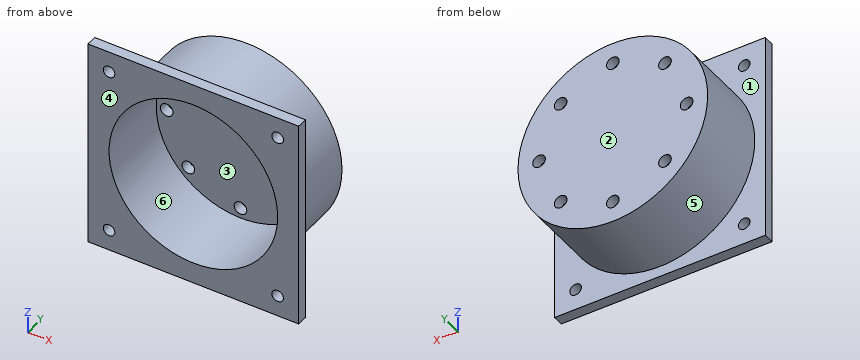
Autodesk Inventor part; units mm, degrees
ref_plane "YZ Plane" through (0, 0, 0) normal (1, 0, 0) x (0, 1, 0)
ref_plane "XZ Plane" through (0, 0, 0) normal (0, 1, 0) x (-1, 0, 0)
ref_plane "XY Plane" through (0, 0, 0) normal (0, 0, 1) x (1, 0, 0)
sketch "Sketch1" plane through (0, 0, 0) normal (0, 1, 0) x (-1, 0, 0)
  line L0 (50, 50) -> (-50, 50)
  line L1 (-50, 50) -> (-50, -50)
  line L2 (-50, -50) -> (50, -50)
  line L3 (50, -50) -> (50, 50)
  circle A0 centre (0, 0) radius 35
  circle A1 centre (40, 40) radius 2.75
  circle A2 centre (-40, 40) radius 2.75
  circle A3 centre (-40, -40) radius 2.75
  circle A4 centre (40, -40) radius 2.75
  point P0 (50, 0)
  point P1 (0, -50)
  dimension "d0" = 100
  dimension "d1" = 100
  dimension "d2" = 70
  dimension "d3" = 5.5
  dimension "d4" = 10
  dimension "d5" = 10
  dimension "d8" = 360
extrude "Extrusion1" add sketch "Sketch1" along normal blind 5
sketch "Sketch2" plane through (0, 0, 0) normal (0, -1, 0) x (1, 0, 0)
  circle A0 centre (0, 0) radius 45
  dimension "d12" = 90
extrude "Extrusion2" cut sketch "Sketch2" against normal blind 10
sketch "Sketch3" plane through (0, 0, 0) normal (0, -1, 0) x (1, 0, 0)
  circle A0 centre (0, 0) radius 45
  circle A1 centre (0, 0) radius 40
  dimension "d15" = 90
  dimension "d16" = 80
extrude "Extrusion3" add sketch "Sketch3" against normal blind 40
sketch "Sketch4" plane through (0, 40, 0) normal (0, 1, 0) x (1, 0, 0)
  circle A0 centre (0, 0) radius 40
extrude "Extrusion4" add sketch "Sketch4" against normal blind 5
sketch "Sketch5" plane through (0, 35, 0) normal (0, -1, 0) x (1, 0, 0)
  circle A0 centre (0, 35) radius 3
  point P0 (0, 0)
  dimension "d21" = 6
  dimension "d22" = 35
extrude "Extrusion5" cut sketch "Sketch5" against normal up to next
pattern_circular "Circular Pattern1" count 8 over 360 about axis through (0, 0, 0) along (0, 1, 0) of "Extrusion5"
properties part number "connector plate"
Could you check a few things on this model? Use its own coordinates, in mm. Face numbers are marked on the shaded views. A direction names the side the tool comes from. Coordinates: 2 decimals unless noted, no trailing zeros. Write each loop counter-clockwise with the first axis right and the second up, starting at its lowest first coordinate (ties: lowest second). Pieces come first, ordered by that corner, then holes. Notation, with made-up numbers: M 7.5,15.25 L 38.5,15.25 A24 cw 38.5,53.25 Z; hole C 74,12 d11. An arc over 180 degrees is marked long. Answer as CSV lines item,"result". Start each with the question number.
1) For the marked faces 1 and 2, which set-ups out of +Z, -Z, +X, -X, +Y, -Y let a thin tool reach every point of the face, with its end or its side?
2) Please list where these lines run through material, in increasing order: line 1 (Z direction, x = 0, y = 38.05); line 2 (Z direction, x = 0, y = 23.5); line 3 (Y direction, x = -2, z = 22). Write a range as from..to.
3) For P1, Ø7, axis at x = 35, z = 0, coming from the -Y side; P2, Ø4, axis at x = -15, y = 23.5, coming from the +Z side; P3, Ø6, axis at x = -18.5, y = 10, coming from the +Z side, each with a flat end and sliding along its axis, tell me the tip position at first contact or that it passes through.
4) We'd pull the mould along Z, two halves only. Please class the marked faces 3, 4, 5 and 6: +Z half, -Z half, draft (parallel to the pull), parting line (faces both ways), or undercut.
5) I want a section at A-A, the plane x = 0. Please give me the cut outline in (y, z).
6) I want a section at D-D, the plane z = -24. Please give me the cut outline in (x, y), and give its area (4 significant figures).
7) I want a section at B-B, the plane z = -35. Please give me the cut outline in (x, y).
8) I want a section at C-C, the plane y = 23. Please give me the cut outline in (x, z).
Data:
1,face 1,"+Y"
1,face 2,"+Z, -Z, +X, -X, +Y"
2,line 1,"z = -45..-38, -32..32, 38..45"
2,line 2,"z = -45..-40, 40..45"
2,line 3,"y = 35..40"
3,P1,"stops at y = 35"
3,P2,"stops at z = 43.08"
3,P3,"stops at z = 42.25"
4,face 3,"undercut"
4,face 4,"draft"
4,face 5,"parting line"
4,face 6,"undercut"
5,outline,"M 0,-50 L 5,-50 L 5,-45 L 40,-45 L 40,-38 L 35,-38 L 35,-40 L 0,-40 Z; M 0,40 L 35,40 L 35,38 L 40,38 L 40,45 L 5,45 L 5,50 L 0,50 Z; M 35,-32 L 40,-32 L 40,32 L 35,32 Z"
6,outline,"M -50,0 L -32,0 L -32,35 L -27.65,35 L -27.65,40 L -38.07,40 L -38.07,5 L -50,5 Z; M -21.84,35 L 21.84,35 L 21.84,40 L -21.84,40 Z; M 27.65,35 L 32,35 L 32,0 L 50,0 L 50,5 L 38.07,5 L 38.07,40 L 27.65,40 Z"
6,area,"866.5 mm^2"
7,outline,"M -50,0 L -19.36,0 L -19.36,35 L -3,35 L -3,40 L -28.28,40 L -28.28,5 L -50,5 Z; M 3,35 L 19.36,35 L 19.36,0 L 50,0 L 50,5 L 28.28,5 L 28.28,40 L 3,40 Z"
8,outline,"C 0,0 d90; hole C 0,0 d80"
